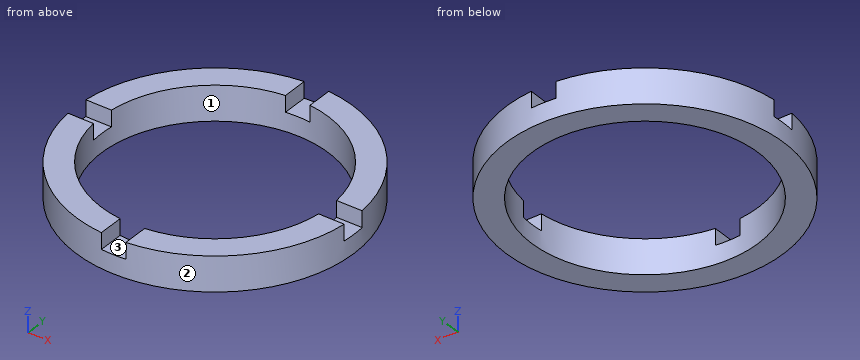
from build123d import *

# Parameters (mm, degrees)
F0_R     = 30
F0_R_2   = 24.5
F1_DEPTH = 7.5
F3_DEPTH = 3.5


with BuildPart() as f1:
    # F0 (on Top) → F1 (new body)
    with BuildSketch(Plane.XY):
        Circle(F0_R)
        Circle(F0_R_2, mode=Mode.SUBTRACT)
    extrude(amount=F1_DEPTH)

    # F2 (on face) → F3 (cut)
    with BuildSketch(Plane.XY.offset(7.5)):
        with BuildLine():
            Line((-2.65, -24.3562620285), (-2.65, -29.8827291257))
            ThreePointArc((-2.65, -29.8827291257), (0, -30), (2.65, -29.8827291257))
            Line((2.65, -29.8827291257), (2.65, -24.3562620285))
            ThreePointArc((2.65, -24.3562620285), (0, -24.5), (-2.65, -24.3562620285))
        make_face()
        with BuildLine():
            ThreePointArc((30, 0), (29.9706679419, 1.3262967671), (29.8827291257, 2.65))
            Line((29.8827291257, 2.65), (24.3562620285, 2.65))
            ThreePointArc((24.3562620285, 2.65), (24.4640391156, 1.3269476821), (24.5, 0))
            ThreePointArc((24.5, 0), (24.4640391156, -1.3269476821), (24.3562620285, -2.65))
            Line((24.3562620285, -2.65), (29.8827291257, -2.65))
            ThreePointArc((29.8827291257, -2.65), (29.9706679419, -1.3262967671), (30, 0))
        make_face()
        with BuildLine():
            ThreePointArc((2.65, 29.8827291257), (0, 30), (-2.65, 29.8827291257))
            Line((-2.65, 29.8827291257), (-2.65, 24.3562620285))
            ThreePointArc((-2.65, 24.3562620285), (0, 24.5), (2.65, 24.3562620285))
            Line((2.65, 24.3562620285), (2.65, 29.8827291257))
        make_face()
        with BuildLine():
            Line((-24.3562620285, 2.65), (-29.8827291257, 2.65))
            ThreePointArc((-29.8827291257, 2.65), (-30, 0), (-29.8827291257, -2.65))
            Line((-29.8827291257, -2.65), (-24.3562620285, -2.65))
            ThreePointArc((-24.3562620285, -2.65), (-24.5, 0), (-24.3562620285, 2.65))
        make_face()
    extrude(amount=-F3_DEPTH, mode=Mode.SUBTRACT)


solid = f1.part
Can you work these out from the model? Positions are in its coordinate system, mm. Face numbers are marked on the shaded views. Coordinates: 2 decimals unless noted, no trailing zeros. Loops run counter-clockwise (first coordinate to the right, second up) from the corner with the lowest first, then second, coordinate; pieces in that order, holes last. Notation, with made-up numbers: M -38,-38.75 L 5,-38.75 A21 cw 5,-20.75 Z; hole C 42.25,13.5 d8. An arc over 180 degrees is marked long. Return JSON: item names as keys, results as strings. Group by question number.
Item 1: I'm going to push flat-ended pins straight in: pin 1 Ø1 at (x, z) = (-27, 5.5) entering from -Y; pin 2 Ø1 at (x, z) = (28, 5.5) entering from +Y; pin 3 Ø4 at (y, z) = (-26.5, 5.5) entering from -X. Where does each tip first touch, or does it pass through?
Item 2: Imagine slicing it at A-A (x = 0). Please give me the cut outline in (y, z).
Item 3: Thinking about a two-plate mould opening in Y: for the marked faces 1, 2 and 3, which applies, released by +Y, released by -Y, zero draft, split by the parting line, or undercut?
Item 4: If I drill on L1, parallel to X at y = 0, z = 3; L2, parallel to Y at x = 26.5, z = 7.25, over which ranges is the centre line in solid material (lowest first)? Write a range as from..to.
Item 5: Imagine slicing it at D-D (y = 26.5). Please give me the cut outline in (x, z).
Item 6: Imagine slicing it at C-C (z = 5). Please give me the cut outline in (x, y), and give its area (3 significant figures).
Verdict:
{
 "1": {"pin 1": "stops at y = -14.06", "pin 2": "stops at y = 11.99", "pin 3": "stops at x = -17.31"},
 "2": {"outline": "M -30,0 L -24.5,0 L -24.5,4 L -30,4 Z; M 24.5,0 L 30,0 L 30,4 L 24.5,4 Z"},
 "3": {"face 1": "undercut", "face 2": "split by the parting line", "face 3": "zero draft"},
 "4": {"L1": "x = -30..-24.5, 24.5..30", "L2": "y = -14.06..-2.65, 2.65..14.06"},
 "5": {"outline": "M -14.06,0 L 14.06,0 L 14.06,7.5 L 2.65,7.5 L 2.65,4 L -2.65,4 L -2.65,7.5 L -14.06,7.5 Z"},
 "6": {"outline": "M -29.88,-2.65 A30 ccw -2.65,-29.88 L -2.65,-24.36 A24.5 cw -24.36,-2.65 Z; M -29.88,2.65 L -24.36,2.65 A24.5 cw -2.65,24.36 L -2.65,29.88 A30 ccw Z; M 2.65,-29.88 A30 ccw 29.88,-2.65 L 24.36,-2.65 A24.5 cw 2.65,-24.36 Z; M 2.65,24.36 A24.5 cw 24.36,2.65 L 29.88,2.65 A30 ccw 2.65,29.88 Z", "area": "825 mm^2"}
}
